Work out the finished part from the listing and answer in its coordinate system (mm). Face numbers are marked on the shaded views. A direction names the side the tool comes from. Coordinates: 2 decimals unless noted, no trailing zeros. Order: outer loops, then holes, each group sorted by start corner. A loop starts at its lowest first (then second) coordinate and runs counter-clockwise, first axis right, second up.
1. A tool of negligible diameter and unlimited length cuts with its end or side. For the marked faces 1, 2, 3, 4 and 5, from which of +Z, -Z, +X, -X, +Y, -Y can it reach the whole face along a straight path? Write none if from no direction.
2. The part is cut by section A-A, the plane z = -7.5. Give the vertices of the cut face in (x, y), then the cut area to 3 significant figures.
3. Determine the mould class of the marked faces 6, 7 and 8 for opening direction Y: +Y half, -Y half, draft (parallel to the pull), parting line (faces both ways), or undercut.
4. The part is cut by section B-B, the plane z = 4.75. Give the vertices of the cut face in (x, y), then the cut area to 3 significant figures.
5. The part is cut by section D-D, the plane y = 35. Give the vertices of the cut face in (x, z).
6. Flat-ended cylindrical pins translate along their axes: pin 1 Ø10 at (x, y) = (7.5, 74.5) entering from -Z; pin 2 Ø5 at (x, y) = (30.5, 7.5) entering from -Z; pin 3 Ø14 at (x, y) = (15.5, 36) entering from -Z; pin 4 Ø1 at (x, y) = (30.5, 61) entering from -Z. Find the tip coordinate at first contact, or state that the pin passes through.
7. Find the intervals of material crossed by probe 1 along Y at (x, z) = (27, -7.5); probe 2 along Y at (x, z) = (32, -5); probe 3 along Z at (x, y) = (30, 19), in increasing order.
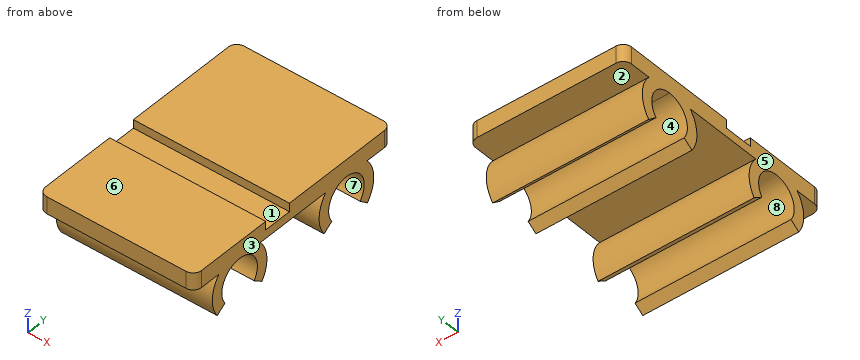
```python
from build123d import *

# Parameters (mm, degrees)
F1_DEPTH = 6
F2_W     = 55
F2_H     = 10
F3_DEPTH = 3
F5_DEPTH = 55


with BuildPart() as f1:
    # F0 (on Top) → F1 (new body)
    with BuildSketch(Plane.XY):
        with BuildLine():
            ThreePointArc((0, 3), (0.87868, 0.87868), (3, 0))
            Line((3, 0), (52, 0))
            ThreePointArc((52, 0), (54.12132, 0.87868), (55, 3))
            Line((55, 3), (55, 80))
            ThreePointArc((55, 80), (54.12132, 82.12132), (52, 83))
            Line((52, 83), (3, 83))
            ThreePointArc((3, 83), (0.87868, 82.12132), (0, 80))
            Line((0, 80), (0, 3))
        make_face()
    extrude(amount=F1_DEPTH)

    # F2 (on face) → F3 (cut)
    with BuildSketch(Plane.XY.offset(6)):
        with Locations((27.5, 35)):
            Rectangle(F2_W, F2_H)
    extrude(amount=-F3_DEPTH, mode=Mode.SUBTRACT)

    # F4 (on face) → F5 (join, through all)
    with BuildSketch(Plane(origin=(0, 0, 0), x_dir=(0, -1, 0), z_dir=(-1, 0, 0))):
        with BuildLine():
            ThreePointArc((-69.745333, -12.320907), (-64.327145, -0.007138), (-57.85636, -11.801823))
            Line((-57.85636, -11.801823), (-54.579751, -14.096129))
            ThreePointArc((-54.579751, -14.096129), (-64.501623, 3.989055), (-72.809511, -14.892058))
            Line((-72.809511, -14.892058), (-69.745333, -12.320907))
        make_face()
        with BuildLine():
            ThreePointArc((-25.14364, -11.801823), (-19, 0), (-12.85636, -11.801823))
            Line((-12.85636, -11.801823), (-9.579751, -14.096129))
            ThreePointArc((-9.579751, -14.096129), (-19, 4), (-28.420249, -14.096129))
            Line((-28.420249, -14.096129), (-25.14364, -11.801823))
        make_face()
    extrude(amount=-F5_DEPTH)


solid = f1.part
```
Geometry says:
1. face 1: +Z, +X, -X
1. face 2: +X, -X, +Y
1. face 3: +Z, -Z, +X, +Y, -Y
1. face 4: +X, -X
1. face 5: +Z, -Z, -X, +Y, -Y
2. outline: (0, 7.5) - (55, 7.5) - (55, 11.5) - (0, 11.5) - close; (0, 26.5) - (55, 26.5) - (55, 30.5) - (0, 30.5) - close; (0, 52.5) - (55, 52.5) - (55, 56.5) - (0, 56.5) - close; (0, 71.5) - (55, 71.5) - (55, 75.5) - (0, 75.5) - close
2. area: 880 mm2
3. face 6: draft
3. face 7: undercut
3. face 8: undercut
4. outline: (0, 3) arc R3 ccw to (3, 0) - (52, 0) arc R3 ccw to (55, 3) - (55, 30) - (0, 30) - close; (0, 40) - (55, 40) - (55, 80) arc R3 ccw to (52, 83) - (3, 83) arc R3 ccw to (0, 80) - close
4. area: 4,010 mm2
5. outline: (0, 0) - (55, 0) - (55, 3) - (0, 3) - close
6. pin 1: stops at z = -14.89
6. pin 2: stops at z = -14.1
6. pin 3: stops at z = -13.18
6. pin 4: stops at z = -0.87
7. probe 1: y = 7.5 to 11.5, 26.5 to 30.5, 52.5 to 56.5, 71.5 to 75.5
7. probe 2: y = 7.78 to 11.93, 26.07 to 30.22, 52.78 to 56.93, 71.07 to 75.22
7. probe 3: z = 0 to 6
